Here's how the part is built. I have some questions about the finished solid (model axes, mm). Face numbers are marked on the shaded views. A direction names the side the tool comes from. Round coordinates to 2 decimals unless told otherwise and drop trailing zeros. Loops run counter-clockwise (first coordinate to the right, second up) from the corner with the lowest first, then second, coordinate; pieces in that order, holes last. Notation, with made-up numbers: M -17.75,-2 L -2.75,-2 A26 cw -2.75,32 Z; hole C 45.25,-18.75 d10. An arc over 180 degrees is marked long. Use a Markdown table: item, result.
from build123d import *

# Parameters (mm, degrees)
SKETCH1_W           = 19
SKETCH1_H           = 10
BOSS_EXTRUDE1_DEPTH = 3
SKETCH2_W           = 3
SKETCH2_H           = 1.5
CUT_EXTRUDE1_DEPTH  = 3
SKETCH3_W           = 3
SKETCH3_H           = 1.5
CUT_EXTRUDE2_DEPTH  = 3
SKETCH5_W           = 5
SKETCH5_H           = 3
CUT_EXTRUDE6_DEPTH  = 3


with BuildPart() as part:
    # Sketch1 → Boss-Extrude1 (new body)
    with BuildSketch(Plane.XY):
        with Locations((3, 9.633458647)):
            Rectangle(SKETCH1_W, SKETCH1_H)
    extrude(amount=BOSS_EXTRUDE1_DEPTH)

    # Sketch2 → Cut-Extrude1 (cut)
    with BuildSketch(Plane.XY.offset(3)):
        with Locations((-5, 11.883458647)):
            Rectangle(SKETCH2_W, SKETCH2_H)
        with Locations((-5, 7.383458647)):
            Rectangle(SKETCH2_W, SKETCH2_H)
    extrude(amount=-CUT_EXTRUDE1_DEPTH, mode=Mode.SUBTRACT)

    # Sketch3 → Cut-Extrude2 (cut)
    with BuildSketch(Plane.XY.offset(3)):
        with Locations((11, 11.883458647)):
            Rectangle(SKETCH3_W, SKETCH3_H)
        with Locations((11, 7.383458647)):
            Rectangle(SKETCH3_W, SKETCH3_H)
    extrude(amount=-CUT_EXTRUDE2_DEPTH, mode=Mode.SUBTRACT)

    # Sketch5 → Cut-Extrude6 (cut)
    with BuildSketch(Plane.XY.offset(3)):
        with Locations((3, 13.133458647)):
            Rectangle(SKETCH5_W, SKETCH5_H)
    extrude(amount=-CUT_EXTRUDE6_DEPTH, mode=Mode.SUBTRACT)


solid = part.part
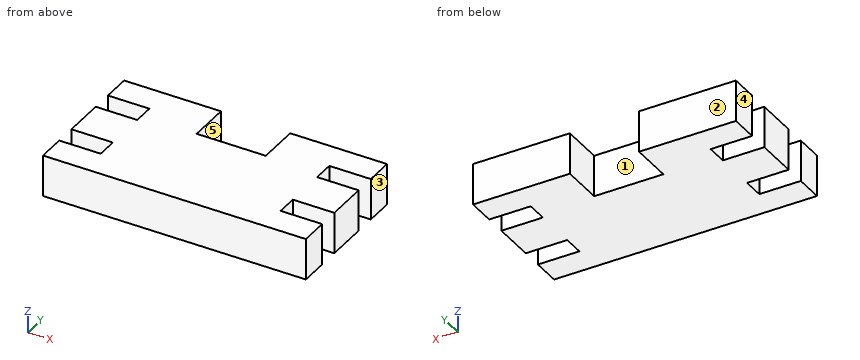
1. For pin 1 Ø3 at (x, y) = (8.5, 9.5) entering from -Z; pin 2 Ø1.5 at (x, z) = (2.5, 2) entering from +Y; pin 3 Ø0.5 at (y, z) = (7.5, 1) entering from +X, each with a flat end and sliding along its axis, tell me the tip position at first contact or that it passes through.
Answer sheet:
| item | result |
|---|---|
| pin 1 | z = 0 |
| pin 2 | y = 11.63 |
| pin 3 | x = 9.5 |
2. Imagine slicing it at A-A, the plane y = 14. Write out the boundary of the cut face in (x, z).
Answer sheet:
| item | result |
|---|---|
| outline | M -6.5,0 L 0.5,0 L 0.5,3 L -6.5,3 Z; M 5.5,0 L 12.5,0 L 12.5,3 L 5.5,3 Z |
3. Imagine slicing it at D-D, the plane y = 7.75. Write out the boundary of the cut face in (x, z), then the cut area to 3 significant figures.
Answer sheet:
| item | result |
|---|---|
| outline | M -3.5,0 L 9.5,0 L 9.5,3 L -3.5,3 Z |
| area | 39.0 mm2 |
4. Imagine slicing it at C-C, the plane x = 0.75. Write out the boundary of the cut face in (y, z).
Answer sheet:
| item | result |
|---|---|
| outline | M 4.63,0 L 11.63,0 L 11.63,3 L 4.63,3 Z |
5. Which directions (+Z, -Z, +X, -X, +Y, -Y) give clear straight access to the entire face, cutting with the end or side of a thin tool? Please do the marked faces 1 and 2.
Answer sheet:
| item | result |
|---|---|
| face 1 | +Z, -Z, +Y |
| face 2 | +Z, -Z, +X, -X, +Y |
6. We'd pull the mould along X, two halves only. Please class the marked faces 3, 4 and 5: +X half, -X half, draft (parallel to the pull), parting line (faces both ways), or undercut.
Answer sheet:
| item | result |
|---|---|
| face 3 | +X half |
| face 4 | -X half |
| face 5 | undercut |
7. I need wall thicknesses on probe 1 along Y at (x, z) = (11.5, 1.15); probe 2 along X at (y, z) = (12.5, 0.1); probe 3 along X at (y, z) = (14.25, 0.3). Which ranges of each line are inside material? Lowest first, please. Write a range as from..to.
Answer sheet:
| item | result |
|---|---|
| probe 1 | 4.63..6.63, 8.13..11.13, 12.63..14.63 |
| probe 2 | -3.5..0.5, 5.5..9.5 |
| probe 3 | -6.5..0.5, 5.5..12.5 |
8. Imagine slicing it at B-B, the plane z = 2.3. Write out the boundary of the cut face in (x, y).
Answer sheet:
| item | result |
|---|---|
| outline | M -6.5,4.63 L 12.5,4.63 L 12.5,6.63 L 9.5,6.63 L 9.5,8.13 L 12.5,8.13 L 12.5,11.13 L 9.5,11.13 L 9.5,12.63 L 12.5,12.63 L 12.5,14.63 L 5.5,14.63 L 5.5,11.63 L 0.5,11.63 L 0.5,14.63 L -6.5,14.63 L -6.5,12.63 L -3.5,12.63 L -3.5,11.13 L -6.5,11.13 L -6.5,8.13 L -3.5,8.13 L -3.5,6.63 L -6.5,6.63 Z |
